```python
from build123d import *

# Parameters (mm, degrees)
SKETCH1_W           = 38.1
SKETCH1_H           = 38.1
SKETCH1_R           = 8.8265
BOSS_EXTRUDE1_DEPTH = 7.62
FILLET1_R           = 2.54
SKETCH2_R           = 2.413
CUT_EXTRUDE1_DEPTH  = 7.62
SKETCH3_R           = 2.413
CUT_EXTRUDE2_DEPTH  = 7.62
SKETCH4_R           = 2.413
CUT_EXTRUDE3_DEPTH  = 39.1


with BuildPart() as part:
    # Sketch1 → Boss-Extrude1 (new body)
    with BuildSketch(Plane.XY):
        Rectangle(SKETCH1_W, SKETCH1_H)
        Circle(SKETCH1_R, mode=Mode.SUBTRACT)
    extrude(amount=BOSS_EXTRUDE1_DEPTH)

    # Fillet1
    fillet1_edges = [part.edges().sort_by_distance(p)[0] for p in [
        (-19.05, 19.05, 3.81),
        (19.05, 19.05, 3.81),
        (19.05, -19.05, 3.81),
        (-19.05, -19.05, 3.81),
    ]]
    fillet(fillet1_edges, radius=FILLET1_R)

    # Sketch2 → Cut-Extrude1 (cut)
    with BuildSketch(Plane.XZ.offset(19.05)):
        with Locations((9.525, 3.81)):
            Circle(SKETCH2_R)
        with Locations((-9.525, 3.81)):
            Circle(SKETCH2_R)
    extrude(amount=-CUT_EXTRUDE1_DEPTH, mode=Mode.SUBTRACT)

    # Sketch3 → Cut-Extrude2 (cut)
    with BuildSketch(Plane(origin=(0, 19.05, 0), x_dir=(1, 0, 0), z_dir=(0, 1, 0))):
        with Locations((-9.525, -3.81)):
            Circle(SKETCH3_R)
        with Locations((9.525, -3.81)):
            Circle(SKETCH3_R)
    extrude(amount=-CUT_EXTRUDE2_DEPTH, mode=Mode.SUBTRACT)

    # Sketch4 → Cut-Extrude3 (cut, through all)
    with BuildSketch(Plane(origin=(0, 19.05, 0), x_dir=(1, 0, 0), z_dir=(0, 1, 0))):
        with Locations((9.525, -3.81)):
            Circle(SKETCH4_R)
        with Locations((-9.525, -3.81)):
            Circle(SKETCH4_R)
    extrude(amount=-CUT_EXTRUDE3_DEPTH, mode=Mode.SUBTRACT)


solid = part.part
```
Work out the finished part from the listing and answer in its coordinate system (mm). Give positions to 0.01 mm unless a question says otherwise; leave off trailing zeros. Write each loop counter-clockwise with the first axis right and the second up, starting at its lowest first coordinate (ties: lowest second). Pieces come first, ordered by that corner, then holes. Notation, with made-up numbers: (44, -18.75) - (49, -18.75) arc R19 cw to (49, 5.25) - close; hole circle Ø5 at (-23.5, -29.5). An arc over 180 degrees is marked (long way). Use one line per item in the form item = value.
1. Determine the mould class of faces 1 (the face through (8, 5, 7.62)), 2 (the face through (11.754, -0.267, 2.886)), 3 (the face through (-6.505, 5.965, 3.757)), 4 (the face through (18.286, 18.326, 3.863)) for opening direction X: released by +X, released by -X, zero draft, split by the parting line, or undercut.
Filled in:
face_1 = zero draft
face_2 = undercut
face_3 = undercut
face_4 = released by +X
2. A cutting plane is placed at B-B (x = 0). Write down the section's boundary in (y, z).
Filled in:
outline = (-19.05, 0) - (-8.83, 0) - (-8.83, 7.62) - (-19.05, 7.62) - close; (8.83, 0) - (19.05, 0) - (19.05, 7.62) - (8.83, 7.62) - close
3. A cutting plane is placed at C-C (z = 6.75). Write down the section's boundary in (x, y).
Filled in:
outline = (-19.05, -16.51) arc R2.54 ccw to (-16.51, -19.05) - (16.51, -19.05) arc R2.54 ccw to (19.05, -16.51) - (19.05, 16.51) arc R2.54 ccw to (16.51, 19.05) - (-16.51, 19.05) arc R2.54 ccw to (-19.05, 16.51) - close; hole circle Ø17.65 at (0, 0)
4. A cutting plane is placed at A-A (y = 6.5). Write down the section's boundary in (x, z) (3 decimals), and give its area (3 significant figures).
Filled in:
outline = (-19.05, 0) - (-5.971, 0) - (-5.971, 7.62) - (-19.05, 7.62) - close; (5.971, 0) - (19.05, 0) - (19.05, 7.62) - (5.971, 7.62) - close; hole circle Ø4.826 at (-9.525, 3.81); hole circle Ø4.826 at (9.525, 3.81)
area = 163 mm^2
5. A cutting plane is placed at D-D (y = 15). Write down the section's boundary in (x, z) (3 decimals), and give its area (3 significant figures).
Filled in:
outline = (-19.05, 0) - (19.05, 0) - (19.05, 7.62) - (-19.05, 7.62) - close; hole circle Ø4.826 at (-9.525, 3.81); hole circle Ø4.826 at (9.525, 3.81)
area = 254 mm^2
6. Consider L1, parallel to X at y = 9, z = 3.81; L2, parallel to Y at x = 0, z = 3; L3, parallel to X at y = 2.5, z = 3.81. Determine where each line is inside the solid, lowest interval first.
Filled in:
L1 = -19.05 to -11.94, -7.11 to 7.11, 11.94 to 19.05
L2 = -19.05 to -8.83, 8.83 to 19.05
L3 = -19.05 to -11.94, 11.94 to 19.05
